Geometry check sheet. Reference: the model listing, model coordinates, mm. Round coordinates to 2 decimals unless told otherwise and drop trailing zeros. Write each loop counter-clockwise with the first axis right and the second up, starting at its lowest first coordinate (ties: lowest second). Pieces come first, ordered by that corner, then holes.
Item 1: Scan lines: probe 1 along Z at (x, y) = (49, -3.35); probe 2 along X at (y, z) = (-0.9, -3); probe 3 along Z at (x, y) = (-16.5, -1.3). Record each from-to range of solid material in increasing order.
Item 2: Depth check by flat-ended pin: P1, Ø1.3, axis at x = -46.41, z = -30.93, coming from the +Y side; P2, Ø6, axis at x = -39.5, z = -40.5, coming from the -Y side. Enter the tip coordinate at first touch or a pass-through.
Item 3: Cross-section at D-D (x = 3). Enter the section's corners in (y, z), then the cut area to 3 significant figures.
Item 4: Cross-section at C-C (z = 49). Enter the section's corners in (x, y).
Item 5: Cross-section at A-A (z = 22). Enter the section's corners in (x, y), then the cut area to 3 significant figures.
Item 6: Cross-section at B-B (x = 49). Enter the section's corners in (y, z).
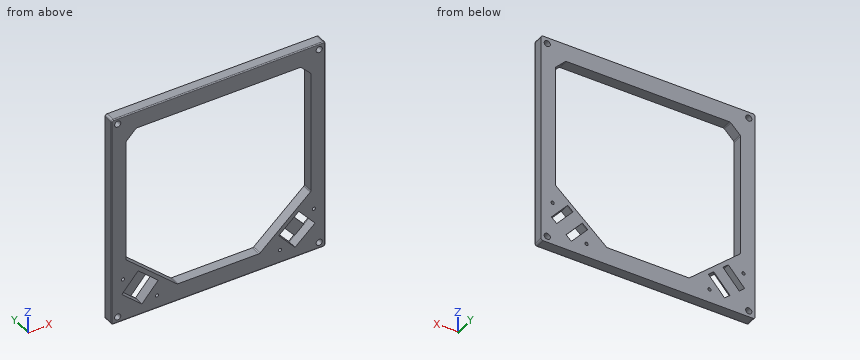
from build123d import *

# Parameters (mm, degrees)
F0_W      = 104
F0_H      = 104
F0_R      = 1.5
F1_DEPTH  = 5
F1_FACE_W = 104
F1_FACE_H = 104
F1_FACE_R = 1.5
F3_DEPTH  = 25
F5_DEPTH  = 4.5
F7_DEPTH  = 2
F8_D      = 1.6
F8_DEPTH  = 15
F9_R      = 1
F10_R     = 0.5


with BuildPart() as f1:
    # F0 (on Front) → F1 (new body)
    with BuildSketch(Plane.XZ):
        Rectangle(F0_W, F0_H)
        with Locations((-49, -49)):
            Circle(F0_R, mode=Mode.SUBTRACT)
        with Locations((49, -49)):
            Circle(F0_R, mode=Mode.SUBTRACT)
        with Locations((-49, 49)):
            Circle(F0_R, mode=Mode.SUBTRACT)
        with Locations((49, 49)):
            Circle(F0_R, mode=Mode.SUBTRACT)
    extrude(amount=F1_DEPTH)

    # F2 (on Front) + F1_face (on face) → F3 (cut)
    with BuildSketch(Plane.XZ):
        Polygon((40, 43.5), (-40, 43.5), (-45, 38.5), (-45, -21.5), (-20, -43.5), (20, -43.5), (45, -21.5), (45, 38.5), align=None)
    with BuildSketch(Plane.XZ.offset(5)):
        Rectangle(F1_FACE_W, F1_FACE_H)
        with Locations((-49, -49)):
            Circle(F1_FACE_R, mode=Mode.SUBTRACT)
        with Locations((49, -49)):
            Circle(F1_FACE_R, mode=Mode.SUBTRACT)
        with Locations((-49, 49)):
            Circle(F1_FACE_R, mode=Mode.SUBTRACT)
        with Locations((49, 49)):
            Circle(F1_FACE_R, mode=Mode.SUBTRACT)
    extrude(amount=F3_DEPTH, mode=Mode.SUBTRACT)

    # F4 (on face) → F5 (cut)
    with BuildSketch(Plane.XZ.offset(5)):
        Polygon((-29.31319, -37.991438), (-39.072465, -29.403275), (-47, -38.411837), (-37.240724, -47), align=None)
        Polygon((47, -38.411837), (39.072465, -29.403275), (29.31319, -37.991438), (37.240724, -47), align=None)
    extrude(amount=-F5_DEPTH, mode=Mode.SUBTRACT)

    # F6 (on face) → F7 (cut)
    with BuildSketch(Plane.XZ.offset(0.5)):
        Polygon((-39.072465, -29.403275), (-47, -38.411837), (-44.372503, -40.724035), (-36.444968, -31.715473), align=None)
        Polygon((-29.31319, -37.991438), (-31.940687, -35.67924), (-39.868222, -44.687802), (-37.240724, -47), align=None)
        Polygon((31.940687, -35.67924), (29.31319, -37.991438), (37.240724, -47), (39.868222, -44.687802), align=None)
        Polygon((36.444968, -31.715473), (44.372503, -40.724035), (47, -38.411837), (39.072465, -29.403275), align=None)
    extrude(amount=-F7_DEPTH, mode=Mode.SUBTRACT)

    # F8
    with Locations(Plane.XZ.offset(5)):
        with Locations((-46.414443, -30.934731), (-29.898746, -45.468544), (29.898746, -45.468544), (46.414443, -30.934731)):
            Hole(F8_D / 2, depth=F8_DEPTH)

    # F9
    f9_edges = [f1.edges().sort_by_distance(p)[0] for p in [
        (-52, -2.5, 52),
        (52, -2.5, 52),
        (52, -2.5, -52),
        (-52, -2.5, -52),
        (-45, -2.5, -21.5),
        (-20, -2.5, -43.5),
        (20, -2.5, -43.5),
        (45, -2.5, -21.5),
        (-45, -2.5, 38.5),
        (-40, -2.5, 43.5),
        (40, -2.5, 43.5),
        (45, -2.5, 38.5),
    ]]
    fillet(f9_edges, radius=F9_R)

    # F10
    f10_edges = [f1.edges().sort_by_distance(p)[0] for p in [
        (0, -5, -52),
    ]]
    fillet(f10_edges, radius=F10_R)


solid = f1.part
Resolved:
1. probe 1: z = -52 to -50.5, -47.5 to 47.5, 50.5 to 52
1. probe 2: x = -52 to -45, 45 to 52
1. probe 3: z = -52 to -43.5, 43.5 to 52
2. P1: passes through
2. P2: stops at y = -0.5
3. outline: (-5, -51.5) arc R0.5 ccw to (-4.5, -52) - (0, -52) - (0, -43.5) - (-5, -43.5) - close; (-5, 43.5) - (0, 43.5) - (0, 52) - (-4.5, 52) arc R0.5 ccw to (-5, 51.5) - close
3. area: 84.9 mm2
4. outline: (-52, -4.5) arc R0.5 ccw to (-51.5, -5) - (-50.5, -5) - (-50.5, 0) - (-52, 0) - close; (-47.5, -5) - (47.5, -5) - (47.5, 0) - (-47.5, 0) - close; (50.5, -5) - (51.5, -5) arc R0.5 ccw to (52, -4.5) - (52, 0) - (50.5, 0) - close
5. outline: (-52, -4.5) arc R0.5 ccw to (-51.5, -5) - (-45, -5) - (-45, 0) - (-52, 0) - close; (45, -5) - (51.5, -5) arc R0.5 ccw to (52, -4.5) - (52, 0) - (45, 0) - close
5. area: 69.9 mm2
6. outline: (-5, -51.5) arc R0.5 ccw to (-4.5, -52) - (0, -52) - (0, -50.5) - (-5, -50.5) - close; (-5, -47.5) - (0, -47.5) - (0, 47.5) - (-5, 47.5) - close; (-5, 50.5) - (0, 50.5) - (0, 52) - (-4.5, 52) arc R0.5 ccw to (-5, 51.5) - close
